from build123d import *

# Parameters (mm, degrees)
SKETCH1_R           = 10
BOSS_EXTRUDE1_DEPTH = 60
SKETCH2_R           = 4
CUT_EXTRUDE1_DEPTH  = 15
BOSS_EXTRUDE2_REACH = 62
CUT_EXTRUDE2_DEPTH  = 20
CHAMFER3_SIZE       = 3
BOSS_EXTRUDE3_START = 18
SKETCH5_R           = 15
BOSS_EXTRUDE3_DEPTH = 3
CHAMFER4_SIZE       = 0.5


with BuildPart() as part:
    # Sketch1 → Boss-Extrude1 (new body)
    with BuildSketch(Plane(origin=(0, 0, 0), x_dir=(1, 0, 0), z_dir=(0, 1, 0))):
        Circle(SKETCH1_R)
    extrude(amount=BOSS_EXTRUDE1_DEPTH)

    # Sketch2 → Cut-Extrude1 (cut)
    with BuildSketch(Plane.XZ):
        Circle(SKETCH2_R)
    extrude(amount=-CUT_EXTRUDE1_DEPTH, mode=Mode.SUBTRACT)

    # Sketch3 → Boss-Extrude2 (add, up to next)
    with BuildSketch(Plane.XZ, mode=Mode.PRIVATE) as boss_extrude2_sk1:
        with BuildLine():
            Line((-2.5, 3.122498999), (-2.5, -3.122498999))
            ThreePointArc((-2.5, -3.122498999), (-4, 0), (-2.5, 3.122498999))
        make_face()
    boss_extrude2_tool1 = extrude(boss_extrude2_sk1.sketch, amount=-BOSS_EXTRUDE2_REACH, mode=Mode.PRIVATE) - part.part
    add(boss_extrude2_tool1.solids().sort_by_distance((-3.110827, 0, 0))[0])

    # Sketch4 → Cut-Extrude2 (cut)
    with BuildSketch(Plane(origin=(0, 60, 0), x_dir=(1, 0, 0), z_dir=(0, 1, 0))):
        with BuildLine():
            Line((-6, 8), (-6, -8))
            ThreePointArc((-6, -8), (-10, 0), (-6, 8))
        make_face()
    extrude(amount=-CUT_EXTRUDE2_DEPTH, mode=Mode.SUBTRACT)

    # Chamfer3
    chamfer3_edges = [part.edges().sort_by_distance(p)[0] for p in [
        (-10, 0, 0),
    ]]
    chamfer(chamfer3_edges, length=CHAMFER3_SIZE)

    # Sketch5 → Boss-Extrude3 (add)
    with BuildSketch(Plane(origin=(0, 0, 0), x_dir=(1, 0, 0), z_dir=(0, 1, 0)).offset(BOSS_EXTRUDE3_START)):
        Circle(SKETCH5_R)
    extrude(amount=BOSS_EXTRUDE3_DEPTH)

    # Chamfer4
    chamfer4_edges = [part.edges().sort_by_distance(p)[0] for p in [
        (-15, 18, 0),
        (-15, 21, 0),
    ]]
    chamfer(chamfer4_edges, length=CHAMFER4_SIZE)


solid = part.part
Can you work these out from the model? Positions are in its coordinate system, mm. A direction names the side the tool comes from. Give positions to 0.01 mm unless a question says otherwise; leave off trailing zeros. Loops run counter-clockwise (first coordinate to the right, second up) from the corner with the lowest first, then second, coordinate; pieces in that order, holes last. Notation, with made-up numbers: (-35, 36) -> (17, 36) arc R18 cw to (17, 67) -> close; hole circle Ø3 at (-23, -37). An arc over 180 degrees is marked (long way). Return JSON: item names as keys, results as strings.
Q1. On a 3-axis mill with a long thin cutter (end or side, diameter ignored), from which of +Z, -Z, +X, -X, +Y, -Y can I reach the whole of each face in a straight line? I mean faces 1 (the face through (-3, 0, 0)), 2 (the face through (-8, 40, 0)), 3 (the face through (1, 15, 0)). Say none if no direction works.
Checks:
{"face 1": "+Z, -Z, +X, -X, -Y", "face 2": "+Z, -Z, -X, +Y", "face 3": "-Y"}
Q2. I want a section at A-A, the plane x = 0. List the corners of the cut face in (y, z) for me, then the cut area to 3 significant figures.
Checks:
{"outline": "(0, -7) -> (3, -10) -> (18, -10) -> (18, -14.5) -> (18.5, -15) -> (20.5, -15) -> (21, -14.5) -> (21, -10) -> (60, -10) -> (60, 10) -> (21, 10) -> (21, 14.5) -> (20.5, 15) -> (18.5, 15) -> (18, 14.5) -> (18, 10) -> (3, 10) -> (0, 7) -> (0, 4) -> (15, 4) -> (15, -4) -> (0, -4) -> close", "area": "1,100 mm2"}
Q3. For pin 1 Ø2 at (x, z) = (2, 0.5) entering from -Y; pin 2 Ø12 at (y, z) = (46, 4) entering from +X; pin 3 Ø6 at (y, z) = (22.5, 6.5) entering from -X, each with a flat end and sliding along its axis, tell me the tip position at first contact or that it passes through.
Checks:
{"pin 1": "stops at y = 15", "pin 2": "stops at x = 10", "pin 3": "stops at x = -14.38"}
Q4. We'd pull the mould along X, two halves only. Please class faces 4 (the face through (9.54, 40.23, -3)), 5 (the face through (3, 21, -10)), 6 (the face through (-2.5, 7, 0)): released by +X, released by -X, zero draft, split by the parting line, or undercut.
Checks:
{"face 4": "split by the parting line", "face 5": "zero draft", "face 6": "undercut"}
Q5. I want a section at C-C, the plane y = 33.5. List the corners of the cut face in (x, z) for me.
Checks:
{"outline": "circle Ø20 at (0, 0)"}
Q6. I need wall thicknesses on probe 1 along Z at (x, y) = (0, 4.25); probe 2 along X at (y, z) = (6.75, 0); probe 3 along Y at (x, z) = (7, 9.5). Which ranges of each line are inside material? Lowest first, please.
Checks:
{"probe 1": "z = -10 to -4, 4 to 10", "probe 2": "x = -10 to -2.5, 4 to 10", "probe 3": "y = 18 to 21"}
Q7. I want a section at B-B, the plane z = 0. List the corners of the cut face in (x, y) for me, then the cut area to 3 significant figures.
Checks:
{"outline": "(-15, 18.5) -> (-14.5, 18) -> (-10, 18) -> (-10, 3) -> (-7, 0) -> (-2.5, 0) -> (-2.5, 15) -> (4, 15) -> (4, 0) -> (7, 0) -> (10, 3) -> (10, 18) -> (14.5, 18) -> (15, 18.5) -> (15, 20.5) -> (14.5, 21) -> (10, 21) -> (10, 60) -> (-6, 60) -> (-6, 40) -> (-10, 40) -> (-10, 21) -> (-14.5, 21) -> (-15, 20.5) -> close", "area": "1,040 mm2"}
